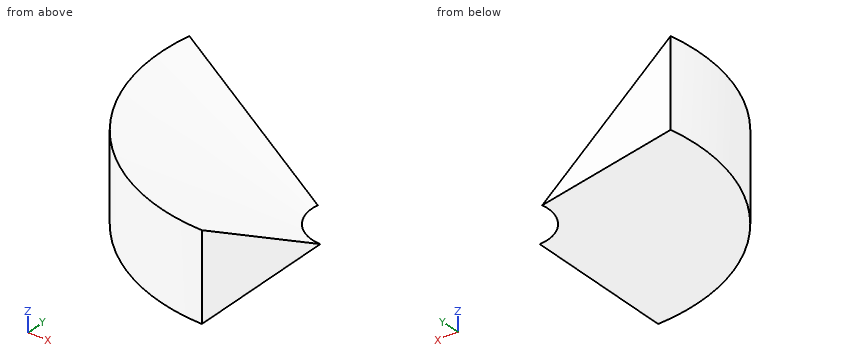
```python
from build123d import *

# Parameters (mm, degrees)
F3_DEPTH = 14.606
F5_DEPTH = 14.606


with BuildPart() as f1:
    # F0 (on Right) → F1 (revolve)
    with BuildSketch(Plane.YZ):
        Polygon((25.4, 14.605), (0, 0), (25.4, 0), align=None)
    revolve(axis=Axis((0, -6.35, 8.989026), (0, 0, 1)))

    # F2 (on Top) → F3 (cut, through all)
    with BuildSketch(Plane.XY):
        Polygon((0, 31.75), (0, -6.35), (0, -41.735239), (38.1, -41.735239), (38.1, -6.35), (38.1, 31.75), align=None)
        Polygon((-6.718058, 31.75), (0, -6.35), (0, 31.75), align=None)
    extrude(amount=F3_DEPTH, mode=Mode.SUBTRACT)

    # F4 (on Top) → F5 (cut, through all)
    with BuildSketch(Plane.XY):
        Polygon((0, -6.35), (0, 27.06758), (-38.1, 27.06758), (-38.1, 0.368058), align=None)
    extrude(amount=F5_DEPTH, mode=Mode.SUBTRACT)


solid = f1.part
```
Model file for the job. Use its own axes, mm. Coordinates: 2 decimals unless noted, no trailing zeros. Order: outer loops, then holes, each group sorted by start corner. A loop starts at its lowest first (then second) coordinate and runs counter-clockwise, first axis right, second up. Notation, with made-up numbers: (46, 63) - (91, 63) arc R8 ccw to (91, 74) - close; hole circle Ø8 at (30.5, 67). An arc over 180 degrees is marked (long way). Return JSON: item names as keys, results as strings. Group by question number.
1) Saw through at B-B, the plane z = 3.75. Write the cut outline in (x, y), plus the area to 3 significant figures.
2) Flat gauge pins, fed straight in: P1, Ø3, axis at x = -20, y = -17, coming from the -Z side; P2, Ø8, axis at y = -25.5, z = 11.5, coming from the -X side; P3, Ø4, axis at y = -25.5, z = 4, coming from the -X side; P4, Ø5, axis at y = -7.5, z = 11.5, coming from the +X side. Where does each tip first touch, or does it go through?
3) Saw through at A-A, the plane z = 5.75. Write the cut outline in (x, y), plus the area to 3 significant figures.
4) Probe line 1 (Y direction, x = -1.5, z = 11.5); line 2 (Z direction, x = -25, y = -24); line 3 (Z direction, x = -28.5, y = -12.5). List the from-to ranges inside material, lowest first. Write a range as from..to.
Values found:
{
 "1": {"outline": "(-31.27, -0.84) arc R31.75 ccw to (0, -38.1) - (0, -19.22) arc R12.87 cw to (-12.68, -4.11) - close", "area": "735 mm²"},
 "2": {"P1": "stops at z = 0", "P2": "stops at x = -27.9", "P3": "stops at x = -26.72", "P4": "stops at x = -21.97"},
 "3": {"outline": "(-31.27, -0.84) arc R31.75 ccw to (0, -38.1) - (0, -22.7) arc R16.35 cw to (-16.1, -3.51) - close", "area": "646 mm²"},
 "4": {"line 1": "y = -38.06..-32.66", "line 2": "z = 0..13.95", "line 3": "z = 0..13.11"}
}
